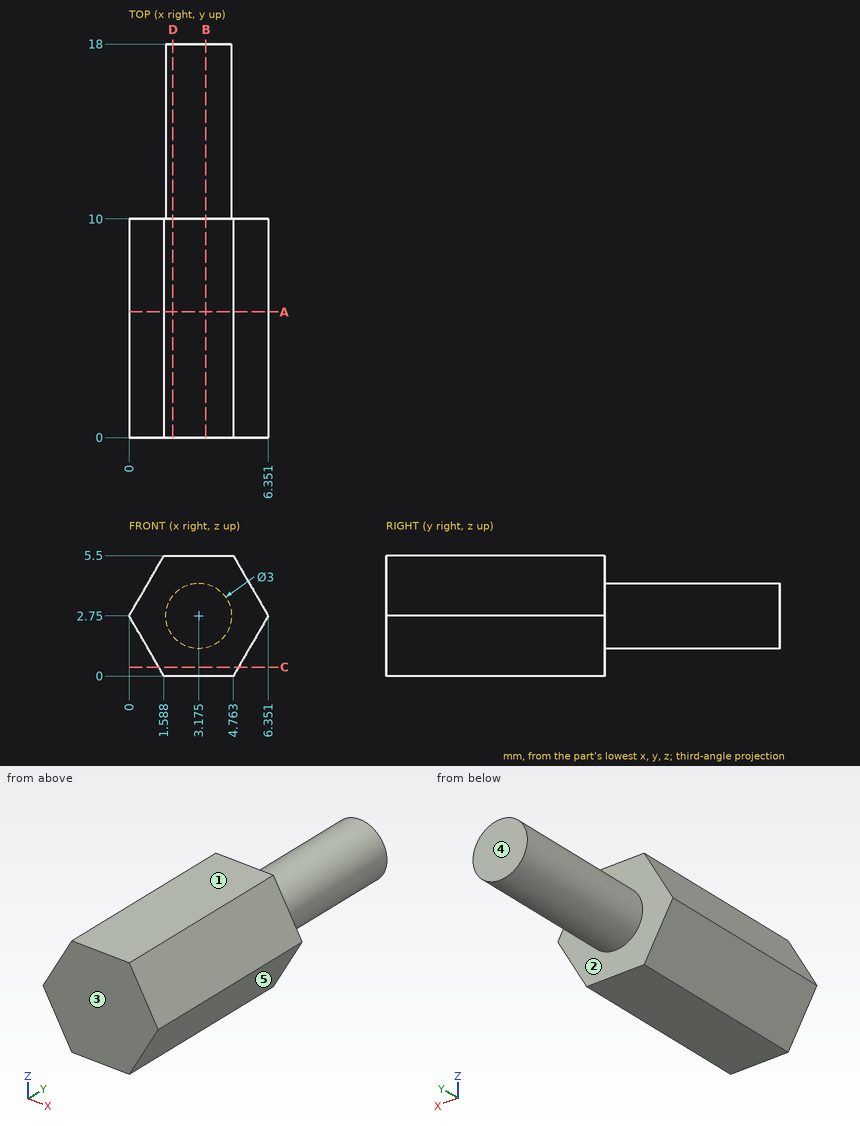
Job drawing, mm, ordinate dimensions from the low corner. One solid piece. A direction names the side the tool comes from. Coordinates: 2 decimals unless noted, no trailing zeros. Order: outer loops, then holes, each group sorted by start corner. A loop starts at its lowest first (then second) coordinate and runs counter-clockwise, first axis right, second up. Notation, with made-up numbers: (54, 42) -> (86, 42) arc R11 cw to (86, 62) -> close; hole circle Ø7 at (-15.5, 67.25). An arc over 180 degrees is marked (long way). Answer in a Markdown table with one row per item. Add a question column.
Q1. Drop flat-ended pins along their axis: pin 1 (2 mm diameter, centred on x = 1.5, y = 15, fed in from +Z); pin 2 (1.5 mm diameter, centred on y = 4.5, z = 1.5, fed in from -X); pin 3 (1.5 mm diameter, centred on x = 1, z = 1, fed in from +Y). Give the stop position or say it passes through.
Q2. Mould opens along Y. For the marked faces 3, 4 and 5 say: +Y half, -Y half, draft (parallel to the pull), parting line (faces both ways), or undercut.
Q3. Wall check: line 1 along Y through (x, z) = (4.5, 5); line 2 along X through (y, z) = (5, 1.3) (1 decimal); line 3 along X through (y, z) = (4.5, 1.2) (1 decimal). Give the ranges that are in metal, low to high. Write a range as [from, to].
Q4. Which spindle directions (+Z, -Z, +X, -X, +Y, -Y) get a long thin tool onto all of the face, cutting with end or side? Do the marked faces 1 and 2. Say none if no direction does.
Q5. Band-saw the part on B-B, the plane x = 3.5. List the corners of the cut face in (y, z) (1 decimal).
Q6. Band-saw the part on A-A, the plane y = 5.75. List the corners of the cut face in (x, z).
Q7. Band-saw the part on C-C, the plane z = 0.4. List the corners of the cut face in (x, y).
Q8. Band-saw the part on D-D, the plane x = 2. List the corners of the cut face in (y, z).
Answers follow:
| question | item | result |
|---|---|---|
| 1 | pin 1 | z = 4.09 |
| 1 | pin 2 | x = 0.29 |
| 1 | pin 3 | y = 10 |
| 2 | face 3 | -Y half |
| 2 | face 4 | +Y half |
| 2 | face 5 | draft |
| 3 | line 1 | [0, 10] |
| 3 | line 2 | [0.8, 5.5] |
| 3 | line 3 | [0.9, 5.5] |
| 4 | face 1 | +Z, +X, -X, +Y, -Y |
| 4 | face 2 | +Y |
| 5 | outline | (0, 0) -> (10, 0) -> (10, 1.3) -> (18, 1.3) -> (18, 4.2) -> (10, 4.2) -> (10, 5.5) -> (0, 5.5) -> close |
| 6 | outline | (0, 2.75) -> (1.59, 0) -> (4.76, 0) -> (6.35, 2.75) -> (4.76, 5.5) -> (1.59, 5.5) -> close |
| 7 | outline | (1.36, 0) -> (4.99, 0) -> (4.99, 10) -> (1.36, 10) -> close |
| 8 | outline | (0, 0) -> (10, 0) -> (10, 1.82) -> (18, 1.82) -> (18, 3.68) -> (10, 3.68) -> (10, 5.5) -> (0, 5.5) -> close |
